Model file for the job. Use its own axes, mm. A direction names the side the tool comes from. Coordinates: 2 decimals unless noted, no trailing zeros. Order: outer loops, then holes, each group sorted by start corner. A loop starts at its lowest first (then second) coordinate and runs counter-clockwise, first axis right, second up. Notation, with made-up numbers: (74, 62) -> (116, 62) arc R31 cw to (116, 92) -> close; hole circle Ø2 at (-25, 33). An arc over 180 degrees is marked (long way). Return JSON: item names as keys, results as strings. Group by question number.
1) Cut at D-D (z = 80.5). Write the cut outline in (x, y).
2) Cut at A-A (x = 49). Write the cut outline in (y, z), and give its area (3 significant figures).
3) Which spindle directions (+Z, -Z, +X, -X, +Y, -Y) get a long thin tool onto all of the face, cutting with end or side? Do faces 4 (the flat face through (-97.606, -3, 34)), 5 (the flat face through (15.225, 57, 71)), 6 (the flat face through (-102, -1, 88.9)). Say none if no direction does.
4) Cut at C-C (z = 12). Write the cut outline in (x, y), and give its area (3 significant figures).
5) Probe line 1 (X direction, y = 43, z = 55); line 2 (Z direction, x = -103, y = 0); line 3 (Y direction, x = -29, z = 36). List the from-to ranges inside material, lowest first.
6) Flat gauge pin, fed straight in: pin 1 (13.5 mm diameter, centred on x = -10, y = -60, fed in from +Z). Where does the tip first touch, or does it go through?
7) Cut at B-B (y = 0). Write the cut outline in (x, z), and give its area (3 significant figures).
8) Pull direction Y, two halves, no side cores. Call faces 1 (the flat face through (52, -1, 88.9)), 2 (the flat face through (-23, 63.081, 44)), 3 (the flat face through (-24, -54.162, 34)): +Y half, -Y half, draft (parallel to the pull), parting line (faces both ways), or undercut.
from build123d import *

# Parameters (mm, degrees)
F0_W     = 176.7475008965
F0_H     = 129.3457597494
F0_W_2   = 149.1751894355
F0_H_2   = 104.7213375568
F1_DEPTH = 88.9
F2_W     = 71.169947274
F2_H     = 34.491557771
F3_DEPTH = 152.4
F4_R     = 12.2849122759
F5_DEPTH = 254


with BuildPart() as f1:
    # F0 (on Top) → F1 (new body)
    with BuildSketch(Plane.XY):
        with Locations((-22.1776217222, -1.5915185213)):
            Rectangle(F0_W, F0_H)
        with Locations((-23.0179391801, -1.8009990454)):
            Rectangle(F0_W_2, F0_H_2, mode=Mode.SUBTRACT)
    extrude(amount=F1_DEPTH)

    # F2 (on face) → F3 (cut)
    with BuildSketch(Plane.XZ.offset(66.264398396)):
        with Locations((-20.3596032225, 71.6542211145)):
            Rectangle(F2_W, F2_H)
    extrude(amount=-F3_DEPTH, mode=Mode.SUBTRACT)

    # F4 (on face) → F5 (cut)
    with BuildSketch(Plane.YZ.offset(66.196128726)):
        with Locations((0, 49.2339283228)):
            Circle(F4_R)
    extrude(amount=-F5_DEPTH, mode=Mode.SUBTRACT)


solid = f1.part
Answers below:
{
 "1": {"outline": "(-110.55, -66.26) -> (-55.94, -66.26) -> (-55.94, -54.16) -> (-97.61, -54.16) -> (-97.61, 50.56) -> (-55.94, 50.56) -> (-55.94, 63.08) -> (-110.55, 63.08) -> close; (15.23, -66.26) -> (66.2, -66.26) -> (66.2, 63.08) -> (15.23, 63.08) -> (15.23, 50.56) -> (51.57, 50.56) -> (51.57, -54.16) -> (15.23, -54.16) -> close"},
 "2": {"outline": "(-66.26, 0) -> (-54.16, 0) -> (-54.16, 88.9) -> (-66.26, 88.9) -> close; (50.56, 0) -> (63.08, 0) -> (63.08, 88.9) -> (50.56, 88.9) -> close", "area": "2,190 mm^2"},
 "3": {"face 4": "+Z, -Z", "face 5": "+Z, +Y, -Y", "face 6": "+Z, +X, -X, +Y, -Y"},
 "4": {"outline": "(-110.55, -66.26) -> (66.2, -66.26) -> (66.2, 63.08) -> (-110.55, 63.08) -> close; hole (-97.61, -54.16) -> (51.57, -54.16) -> (51.57, 50.56) -> (-97.61, 50.56) -> close", "area": "7,240 mm^2"},
 "5": {"line 1": "x = -110.55 to -97.61, 51.57 to 66.2", "line 2": "z = 0 to 36.95, 61.52 to 88.9", "line 3": "y = -66.26 to -54.16, 50.56 to 63.08"},
 "6": {"pin 1": "stops at z = 54.41"},
 "7": {"outline": "(-110.55, 0) -> (-97.61, 0) -> (-97.61, 36.95) -> (-110.55, 36.95) -> close; (-110.55, 61.52) -> (-97.61, 61.52) -> (-97.61, 88.9) -> (-110.55, 88.9) -> close; (51.57, 0) -> (66.2, 0) -> (66.2, 36.95) -> (51.57, 36.95) -> close; (51.57, 61.52) -> (66.2, 61.52) -> (66.2, 88.9) -> (51.57, 88.9) -> close", "area": "1,770 mm^2"},
 "8": {"face 1": "draft", "face 2": "+Y half", "face 3": "undercut"}
}
